Part model, mm, in its own coordinate system. A direction names the side the tool comes from. Coordinates: 2 decimals unless noted, no trailing zeros. Order: outer loops, then holes, each group sorted by start corner. A loop starts at its lowest first (then second) coordinate and runs counter-clockwise, first axis right, second up. Notation, with made-up numbers: M 45,1 L 51,1 A18 ccw 51,11 Z; hole C 15,-20 d11. An arc over 180 degrees is marked long. Answer in a Markdown table with one row per item. Add a question column.
from build123d import *

# Parameters (mm, degrees)
BOSS_EXTRUDE1_DEPTH = 15
FILLET1_R           = 7
CUT_EXTRUDE1_DEPTH  = 46.581927456
FILLET2_R           = 3


with BuildPart() as part:
    # Sketch1 → Boss-Extrude1 (new body)
    with BuildSketch(Plane.XY):
        with BuildLine():
            Line((81.814228499, 422.253610621), (101.396155955, 422.253610621))
            ThreePointArc((101.396155955, 422.253610621), (112.002757673, 426.647008903), (116.396155955, 437.253610621))
            Line((116.396155955, 437.253610621), (116.396155955, 525.576232013))
            Line((116.396155955, 525.576232013), (128.396155955, 525.576232013))
            Line((128.396155955, 525.576232013), (128.396155955, 437.253610621))
            ThreePointArc((128.396155955, 437.253610621), (121.073825485, 419.575941091), (103.396155955, 412.253610621))
            Line((103.396155955, 412.253610621), (81.814228499, 412.253610621))
            Line((81.814228499, 412.253610621), (81.814228499, 422.253610621))
        make_face()
    extrude(amount=-BOSS_EXTRUDE1_DEPTH)

    # Fillet1
    fillet1_edges = [part.edges().sort_by_distance(p)[0] for p in [
        (122.396155955, 525.576232013, -15),
        (122.396155955, 525.576232013, 0),
    ]]
    fillet(fillet1_edges, radius=FILLET1_R)

    # Sketch2 → Cut-Extrude1 (cut)
    with BuildSketch(Plane(origin=(128.396155955, 0, 0), x_dir=(0, 0, -1), z_dir=(1, 0, 0))):
        Polygon((0, 419.753610621), (7.5, 412.253610621), (15, 419.753610621), (15, 408.691340296), (0, 408.691340296), align=None)
    extrude(amount=-CUT_EXTRUDE1_DEPTH, mode=Mode.SUBTRACT)

    # Fillet2
    fillet2_edges = [part.edges().sort_by_distance(p)[0] for p in [
        (101.531977763, 419.753610621, -15),
        (101.531977763, 419.753610621, 0),
    ]]
    fillet(fillet2_edges, radius=FILLET2_R)


solid = part.part
(1) Drop flat-ended pins along their axis: P1, Ø6, axis at x = 107.5, z = -1.5, coming from the -Y side; P2, Ø4.5, axis at y = 467.5, z = -4.5, coming from the -X side. Give the stop position or say it passes through.
(2) Wall check: line 1 (X direction, y = 470, z = -6.5); line 2 (Z direction, x = 126, y = 519); line 3 (Y direction, x = 124, z = -14). Give the ranges that are in metal, low to high.
(3) Slice it at C-C (y = 501.5). List the corners of the cut face in (x, z), and give its area (3 significant figures).
(4) 3-axis set-ups, long thin cutter, end or side, ignore diameter. For faces 1 (the flat face through (116.396, 481, -7)), 2 (the flat face through (97.068, 415.518, -10.764)): which of +Z, -Z, +X, -X, +Y, -Y reach the whole face in a straight line?
(5) Slice it at B-B (x = 112). List the corners of the cut face in (y, z).
(6) Slice it at A-A (z = -11). List the corners of the cut face in (x, y).
(7) Slice it at D-D (x = 96.5). List the corners of the cut face in (y, z).
Computed:
| question | item | result |
|---|---|---|
| 1 | P1 | stops at y = 415.25 |
| 1 | P2 | stops at x = 116.4 |
| 2 | line 1 | x = 116.4 to 128.4 |
| 2 | line 2 | z = -14.99 to -0.01 |
| 2 | line 3 | y = 423.09 to 522.18 |
| 3 | outline | M 116.4,-15 L 128.4,-15 L 128.4,0 L 116.4,0 Z |
| 3 | area | 180 mm^2 |
| 4 | face 1 | +Z, -Z, -X, +Y |
| 4 | face 2 | -Z, +X, -X, -Y |
| 5 | outline | M 413.78,-9.03 L 418.87,-14.12 A3 ccw 421,-15 L 426.64,-15 L 426.64,0 L 421,0 A3 ccw 418.87,-0.88 L 413.78,-5.97 Z |
| 6 | outline | M 81.81,415.75 L 116.15,415.75 A25 ccw 128.4,437.25 L 128.4,524.9 L 116.4,524.9 L 116.4,437.25 A15 cw 101.4,422.25 L 81.81,422.25 Z |
| 7 | outline | M 412.25,-7.5 L 418.87,-14.12 A3 ccw 421,-15 L 422.25,-15 L 422.25,0 L 421,0 A3 ccw 418.87,-0.88 Z |
